from build123d import *

# Parameters (mm, degrees)
SKETCH_1_R = 0.75
SKETCH_1_W = 1.8
SKETCH_1_H = 3


with BuildPart() as part:
    # Эскиз1 → Повернуть1 (revolve)
    with BuildSketch(Plane(origin=(0, 0, 0), x_dir=(1, 0, 0), z_dir=(0, 1, 0)), mode=Mode.PRIVATE) as revolve_1_sk:
        with Locations((0, 26.85)):
            Circle(SKETCH_1_R)
        Polygon((-3.5, 26.85), (3.5, 26.85), (3.5, 29.75), (0.5, 31.75), (-0.5, 31.75), (-3.5, 29.75), align=None)
        with BuildLine():
            Line((-0.75, 26.85), (0, 26.85))
            Line((0, 26.85), (0.75, 26.85))
            ThreePointArc((0.75, 26.85), (0, 27.6), (-0.75, 26.85))
        make_face()
        with BuildLine():
            ThreePointArc((-0.75, 26.85), (-0.530330086, 26.319669914), (0, 26.1))
            Line((0, 26.1), (0, 26.85))
            Line((0, 26.85), (-0.75, 26.85))
        make_face()
        with BuildLine():
            Line((0, 26.85), (0, 26.1))
            ThreePointArc((0, 26.1), (0.530330086, 26.319669914), (0.75, 26.85))
            Line((0.75, 26.85), (0, 26.85))
        make_face()
        Polygon((-4.5, 29.083333333), (-4.5, 23.85), (-3.5, 23.85), (-3.5, 26.85), (-3.5, 29.75), align=None)
        with Locations((-2.6, 25.35)):
            Rectangle(SKETCH_1_W, SKETCH_1_H)
        with Locations((2.6, 25.35)):
            Rectangle(SKETCH_1_W, SKETCH_1_H)
    revolve(revolve_1_sk.sketch.rotate(Axis((0, 0, 0), (1, 0, 0)), 180), axis=Axis((0, 0, 0), (1, 0, 0)))


solid = part.part
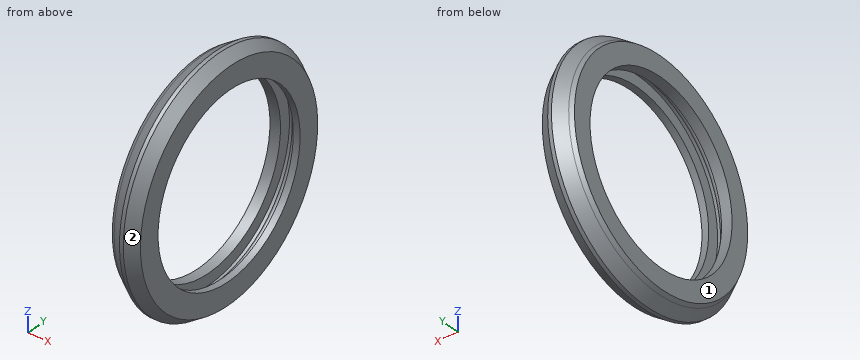
Input: part model. Units: mm. Frame: model coordinates. Face numbers are marked on the shaded views. Give positions to 0.01 mm unless a question says otherwise; leave off trailing zeros. Write each loop counter-clockwise with the first axis right and the second up, starting at its lowest first coordinate (ties: lowest second). Pieces come first, ordered by that corner, then holes.
Q1. Material intervals for probe 1 along X at (y, z) = (24, -3.5); probe 2 along Z at (x, y) = (-1.75, -9); probe 3 along Y at (x, z) = (2.75, 13.5), sorted ascending.
Q2. Pull-direction query (Z, two-part tool) for the marked faces 1 and 2; classes: pulls with the +Z half, pulls with the -Z half, needs draft (parallel to the pull), parting line crosses it, or undercut.
Q3. First-contact query: P1, Ø1.5, axis at x = 1.5, z = 3, coming from the -Y side; P2, Ø2, axis at x = 1.5, y = 20, coming from the -Z side; P3, Ø4, axis at x = 1, y = 11.5, coming from the +Z side. Flat tips, straight axial feed; report the tip coordinate or a pass-through.
Q4. Section A-A, the plane x = -2.75. Output: boundary loops of the cut face in (y, z).
Filled in:
1. probe 1: x = -4.5 to -1.7, 1.7 to 3.5
1. probe 2: z = -29.58 to -22.09, 22.09 to 29.58
1. probe 3: y = -27.07 to -19.66, 19.66 to 27.07
2. face 1: needs draft
2. face 2: parting line crosses it
3. P1: stops at y = -31.45
3. P2: stops at z = -24.97
3. P3: stops at z = 30.28
4. outline: circle Ø60.5 at (0, 0); hole circle Ø47.7 at (0, 0)
